Drawing for the job (mm, zero at the part's lowest x, y, z). A direction names the side the tool comes from. Give positions to 0.01 mm unless a question says otherwise; leave off trailing zeros. Order: outer loops, then holes, each group sorted by start corner. A loop starts at its lowest first (then second) coordinate and runs counter-clockwise, first axis right, second up. Notation, with made-up numbers: (77.5, 47.25) - (126.5, 47.25) arc R28 ccw to (126.5, 69.25) - close; hole circle Ø10 at (70.25, 54.25). An arc over 180 degrees is marked (long way). Use CSV: the item, a comma, the result in double quotes. Start each with the question number.
(1) Tool access for the marked faces 1 and 2: list every direction of +Z, -Z, +X, -X, +Y, -Y with a clear straight run to the whole face (end or side of a thin tool).
(2) Band-saw the part on D-D, the plane y = 2. Give the cut face in (x, z) (1 decimal).
(3) Drop flat-ended pins along their axis: pin 1 Ø1 at (y, z) = (4, 3) entering from -X (3 decimals); pin 2 Ø8.5 at (x, y) = (41.5, 17) entering from -Z. Give the stop position or say it passes through.
(4) Band-saw the part on B-B, the plane z = 5. Count the separate pieces of the cut face and the enclosed holes in it, then the cut area to 3 significant figures.
(5) Pull direction Y, two halves, no side cores. Call the marked faces 3, 4 and 5: +Y half, -Y half, draft (parallel to the pull), parting line (faces both ways), or undercut.
(6) Band-saw the part on A-A, the plane z = 8.75. Give the cut face in (x, y) (1 decimal).
(7) Probe L1, parallel to Y at x = 45, z = 3 (1 decimal); L2, parallel to Z at x = 57, y = 15.5 (1 decimal); L3, parallel to Y at x = 55, z = 10.25. List the from-to ranges inside material, lowest first.
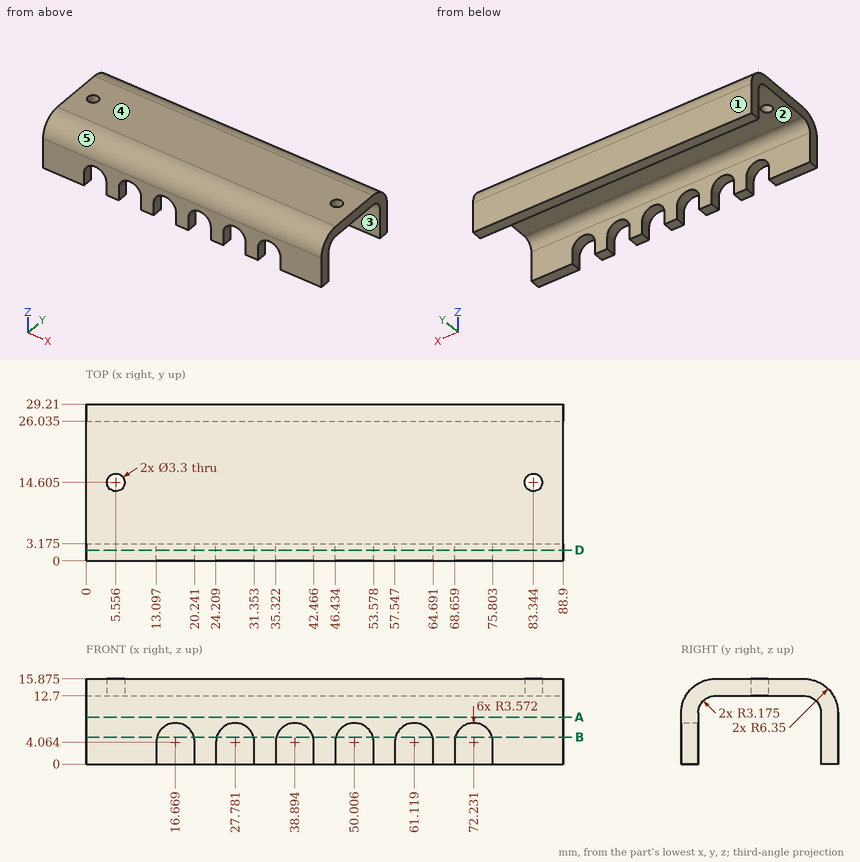
Answer block:
1,face 1,"+Z, -Z, +X, -X, +Y"
1,face 2,"-Z, +X, -X"
2,outline,"(0, 0) - (13.1, 0) - (13.1, 4.1) arc R3.6 cw to (20.2, 4.1) - (20.2, 0) - (24.2, 0) - (24.2, 4.1) arc R3.6 cw to (31.4, 4.1) - (31.4, 0) - (35.3, 0) - (35.3, 4.1) arc R3.6 cw to (42.5, 4.1) - (42.5, 0) - (46.4, 0) - (46.4, 4.1) arc R3.6 cw to (53.6, 4.1) - (53.6, 0) - (57.5, 0) - (57.5, 4.1) arc R3.6 cw to (64.7, 4.1) - (64.7, 0) - (68.7, 0) - (68.7, 4.1) arc R3.6 cw to (75.8, 4.1) - (75.8, 0) - (88.9, 0) - (88.9, 14.2) - (0, 14.2) - close"
3,pin 1,"passes through"
3,pin 2,"stops at z = 12.7"
4,separate pieces,"8"
4,enclosed holes,"0"
4,area,"433 mm2"
5,face 3,"undercut"
5,face 4,"draft"
5,face 5,"-Y half"
6,outline,"(0, 0) - (88.9, 0) - (88.9, 3.2) - (0, 3.2) - close; (0, 26) - (88.9, 26) - (88.9, 29.2) - (0, 29.2) - close"
7,L1,"y = 0 to 3.2, 26 to 29.2"
7,L2,"z = 12.7 to 15.9"
7,L3,"y = 0.04 to 3.26, 25.95 to 29.17"
